Geometry: see drawing. Coordinates: mm, zero at the bounding-box minimum. A direction names the side the tool comes from. Give positions to 0.01 mm unless a question says otherwise; leave off trailing zeros. Write each loop counter-clockwise with the first axis right and the second up, starting at its lowest first coordinate (ties: lowest second). Pieces come first, ordered by that corner, then holes.
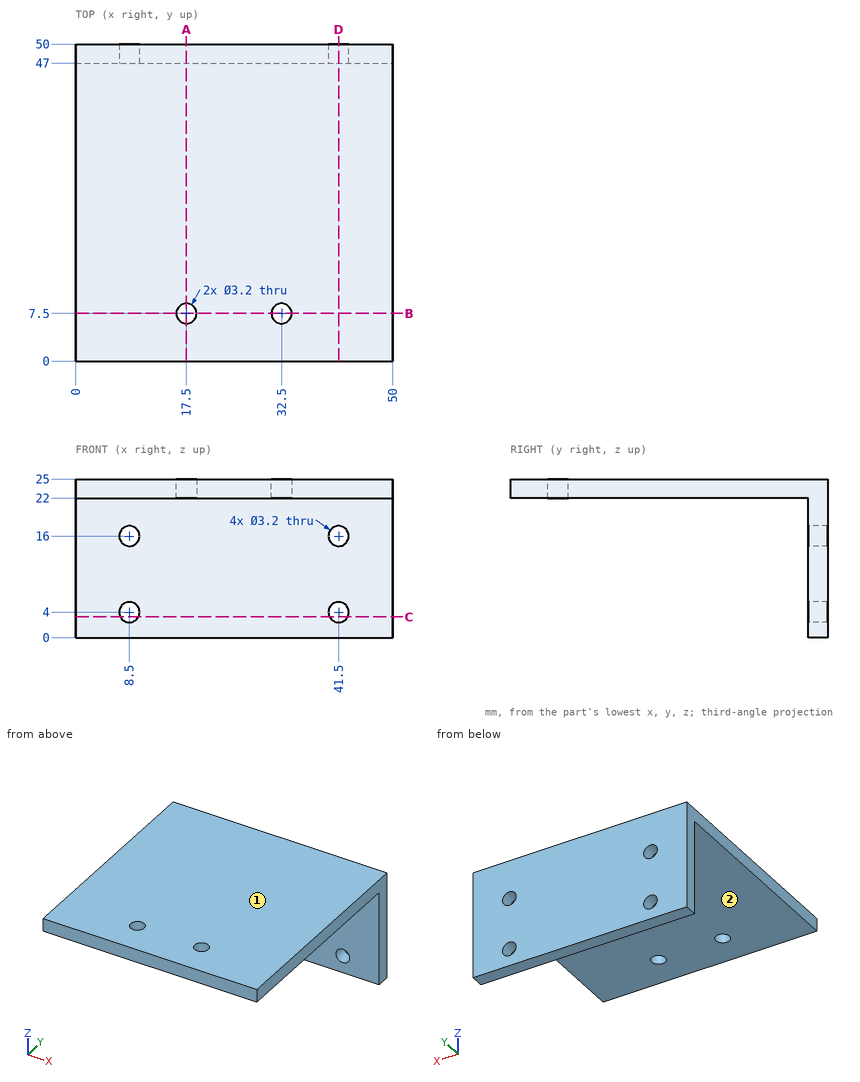
Q1. Section C-C, the plane z = 3.25. Return the cut outline in (x, y).
Q2. Access query for the marked faces 1 and 2. Directions: +Z, -Z, +X, -X, +Y, -Y. A direction counts if a zero-diameter tool reaches every point of the face in a straight line with its end or side. Return the directions, or none.
Q3. Material intervals for line 1 along Z through (x, y) = (8.5, 47.65); line 2 along Y through (x, z) = (32.5, 23.85); line 3 along Z through (x, y) = (30.5, 10), sorted ascending.
Q4. Pin query (flat end, axial travel): pin 1 (1.9 mm diameter, centred on x = 17.5, y = 7.5, fed in from +Z); pin 2 (6 mm diameter, centred on x = 16, y = 6, fed in from -Z). Return the tip coordinate at first contact, or that it passes through.
Q5. Section D-D, the plane x = 41.5. Return the cut outline in (y, z).
Q6. Section A-A, the plane x = 17.5. Return the cut outline in (y, z).
Q7. Section B-B, the plane y = 7.5. Return the cut outline in (x, z).
Solutions:
1. outline: (0, 47) - (7.09, 47) - (7.09, 50) - (0, 50) - close; (9.91, 47) - (40.09, 47) - (40.09, 50) - (9.91, 50) - close; (42.91, 47) - (50, 47) - (50, 50) - (42.91, 50) - close
2. face 1: +Z, +X, -X, +Y, -Y
2. face 2: -Z, +X, -X, -Y
3. line 1: z = 0 to 2.4, 5.6 to 14.4, 17.6 to 25
3. line 2: y = 0 to 5.9, 9.1 to 50
3. line 3: z = 22 to 25
4. pin 1: passes through
4. pin 2: stops at z = 22
5. outline: (0, 22) - (47, 22) - (47, 17.6) - (50, 17.6) - (50, 25) - (0, 25) - close; (47, 0) - (50, 0) - (50, 2.4) - (47, 2.4) - close; (47, 5.6) - (50, 5.6) - (50, 14.4) - (47, 14.4) - close
6. outline: (0, 22) - (5.9, 22) - (5.9, 25) - (0, 25) - close; (9.1, 22) - (47, 22) - (47, 0) - (50, 0) - (50, 25) - (9.1, 25) - close
7. outline: (0, 22) - (15.9, 22) - (15.9, 25) - (0, 25) - close; (19.1, 22) - (30.9, 22) - (30.9, 25) - (19.1, 25) - close; (34.1, 22) - (50, 22) - (50, 25) - (34.1, 25) - close
